Geometry: final body of the model. Coordinates: model frame, mm. Face numbers are marked on the shaded views. A direction names the side the tool comes from. Coordinates: 2 decimals unless noted, no trailing zeros. Loops run counter-clockwise (first coordinate to the right, second up) from the corner with the lowest first, then second, coordinate; pieces in that order, holes last. Notation, with made-up numbers: (-39.75, 38.25) - (-33.75, 38.25) arc R18 ccw to (-33.75, 73.25) - close; hole circle Ø6 at (80.5, -7.5). An arc over 180 degrees is marked (long way). Answer in a Markdown table with one row per item.
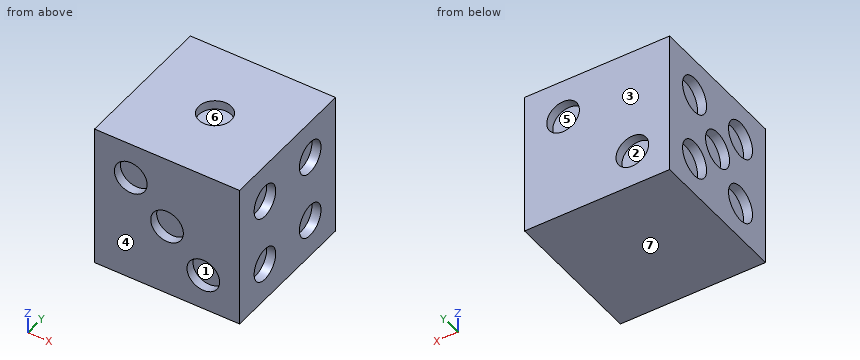
Autodesk Fusion 360 part; units mm, degrees
sketch "Sketch1" plane through (0, 0, 0) normal (0, 0, 1) x (1, 0, 0) in component "Component"
  line L0 (50.8, -50.8) -> (-50.8, -50.8)
  line L1 (-50.8, -50.8) -> (-50.8, 50.8)
  line L2 (-50.8, 50.8) -> (50.8, 50.8)
  line L3 (50.8, 50.8) -> (50.8, -50.8)
  line L4 (50.8, -50.8) -> (-50.8, 50.8) construction
  line L5 (-50.8, -50.8) -> (50.8, 50.8) construction
  dimension "d1" = 101.6
  dimension "d2" = 101.6
extrude "Extrude1" add sketch "Sketch1" along normal mid plane 101.6 in component "Component"
sketch "Sketch2" plane through (0, 0, 50.8) normal (0, 0, 1) x (-1, 0, 0) in component "Component"
  line L0 (-50.8, -50.8) -> (50.8, -50.8)
  line L1 (50.8, -50.8) -> (50.8, 50.8)
  line L2 (50.8, 50.8) -> (-50.8, 50.8)
  line L3 (-50.8, 50.8) -> (-50.8, -50.8)
  circle A0 centre (0, 0) radius 11.43
  dimension "d5" = 22.86
extrude "Extrude2" cut sketch "Sketch2" against normal blind 6.35 contours A0 in component "Component"
sketch "Sketch3" plane through (0, -50.8, 0) normal (0, -1, 0) x (1, 0, 0) in component "Component"
  line L0 (50.8, -50.8) -> (50.8, 50.8)
  line L1 (50.8, 50.8) -> (-50.8, 50.8)
  line L2 (-50.8, 50.8) -> (-50.8, -50.8)
  line L3 (-50.8, -50.8) -> (50.8, -50.8)
  circle A0 centre (0, 0) radius 11.43
  line L4 (-50.8, 50.8) -> (0, 0)
  line L5 (0, 0) -> (50.8, -50.8)
  circle A1 centre (-25.4, 25.4) radius 11.43
  circle A2 centre (25.4, -25.4) radius 11.43
  dimension "d8" = 22.86
  dimension "d9" = 22.86
  dimension "d10" = 22.86
extrude "Extrude3" cut sketch "Sketch3" against normal blind 6.35 contours L5 A2 | L5 A2 | L4 A1 | L4 A1 | A0 L4 L5 | A0 L4 L5 in component "Component"
sketch "Sketch4" plane through (50.8, 0, 0) normal (1, 0, 0) x (0, 1, 0) in component "Component"
  line L0 (50.8, -50.8) -> (50.8, 50.8)
  line L1 (50.8, 50.8) -> (-50.8, 50.8)
  line L2 (-50.8, 50.8) -> (-50.8, -50.8)
  line L3 (-50.8, -50.8) -> (50.8, -50.8)
  line L4 (-50.8, 50.8) -> (50.8, -50.8)
  line L5 (-50.8, -50.8) -> (50.8, 50.8) construction
  circle A0 centre (-23.9624, 23.9624) radius 11.43
  circle A1 centre (23.9624, 23.9624) radius 11.43
  circle A2 centre (-23.9624, -23.9624) radius 11.43
  circle A3 centre (23.9624, -23.9624) radius 11.43
  dimension "d13" = 22.86
extrude "Extrude4" cut sketch "Sketch4" against normal blind 6.35 contours L4 A3 | L4 A3 | L4 A0 | L4 A0 | A1 | A2 in component "Component"
sketch "Sketch5" plane through (0, 50.8, 0) normal (0, 1, 0) x (-1, 0, 0) in component "Component"
  line L0 (50.8, -50.8) -> (50.8, 50.8)
  line L1 (50.8, 50.8) -> (-50.8, 50.8)
  line L2 (-50.8, 50.8) -> (-50.8, -50.8)
  line L3 (-50.8, -50.8) -> (50.8, -50.8)
  line L4 (-50.8, 50.8) -> (50.8, -50.8)
  circle A0 centre (24.6983, -24.6983) radius 11.43
  circle A1 centre (-23.7784, 23.7784) radius 11.43
  dimension "d16" = 22.86
extrude "Extrude5" cut sketch "Sketch5" against normal blind 6.35 contours L4 A0 | L4 A0 | L4 A1 | L4 A1 in component "Component"
sketch "Sketch6" plane through (-50.8, 0, 0) normal (-1, 0, 0) x (0, -1, 0) in component "Component"
  line L0 (50.8, -50.8) -> (50.8, 50.8)
  line L1 (50.8, 50.8) -> (-50.8, 50.8)
  line L2 (-50.8, 50.8) -> (-50.8, -50.8)
  line L3 (-50.8, -50.8) -> (50.8, -50.8)
  line L4 (-50.8, 50.8) -> (50.8, -50.8)
  line L5 (-50.8, -50.8) -> (50.8, 50.8)
  circle A0 centre (0, 0) radius 12.7
  circle A1 centre (-24.3304, 24.3304) radius 12.7
  circle A2 centre (24.3304, 24.3304) radius 12.7
  circle A3 centre (-24.3304, -24.3304) radius 12.7
  circle A4 centre (24.3304, -24.3304) radius 12.7
  dimension "d19" = 25.4
extrude "Extrude6" cut sketch "Sketch6" against normal blind 6.35 contours L4 A4 | L4 A4 | L5 A2 | L5 A2 | L5 A3 | L5 A3 | L4 A1 | L4 A1 | L4 L5 A0 | L4 L5 A0 | L4 L5 A0 | L4 L5 A0 in component "Component"
sketch "Sketch7" plane through (0, 0, -50.8) normal (0, 0, -1) x (1, 0, 0) in component "Component"
  line L0 (-50.8, -50.8) -> (50.8, -50.8)
  line L1 (50.8, -50.8) -> (50.8, 50.8)
  line L2 (50.8, 50.8) -> (-50.8, 50.8)
  line L3 (-50.8, 50.8) -> (-50.8, -50.8)
sketch "Sketch8" plane through (0, 50.8, 0) normal (0, 1, 0) x (-1, 0, 0) in component "Component"
  circle A0 centre (24.6983, -24.6983) radius 11.43
  circle A1 centre (-23.7784, 23.7784) radius 11.43
  line L0 (50.8, -50.8) -> (50.8, 50.8)
  line L1 (50.8, 50.8) -> (-50.8, 50.8)
  line L2 (-50.8, 50.8) -> (-50.8, -50.8)
  line L3 (-50.8, -50.8) -> (50.8, -50.8)
sketch "Sketch10" plane through (0, 0, -50.8) normal (0, 0, -1) x (1, 0, 0) in component "Component"
component "Component" placed x (1, 0, 0) y (0, 1, 0) z (0, 0, 1) at (0, 0, 0)
equation "d1 = dicesize"
equation "d2 = dicesize"
equation "d5 = Divotsize"
equation "d8 = Divotsize"
equation "d9 = Divotsize"
equation "d10 = Divotsize"
equation "d13 = Divotsize"
equation "d16 = Divotsize"
equation "dicesize = 4 in"
equation "Divotsize = 0.9 in"
equation "diceDepth = 0.25 in"
(1) Pull-direction query (Z, two-part tool) for the marked faces 4, 5, 6 and 7; classes: pulls with the +Z half, pulls with the -Z half, needs draft (parallel to the pull), parting line crosses it, or undercut.
Verdict:
| item | result |
|---|---|
| face 4 | needs draft |
| face 5 | undercut |
| face 6 | pulls with the +Z half |
| face 7 | pulls with the -Z half |
(2) Cut plane A-A on y = 0. Output: boundary loops of the cut face in (x, z), then the cut area to 3 significant figures.
Verdict:
| item | result |
|---|---|
| outline | (-50.8, -50.8) - (50.8, -50.8) - (50.8, 50.8) - (11.43, 50.8) - (11.43, 44.45) - (-11.43, 44.45) - (-11.43, 50.8) - (-50.8, 50.8) - (-50.8, 12.7) - (-44.45, 12.7) - (-44.45, -12.7) - (-50.8, -12.7) - close |
| area | 10,000 mm² |
(3) Cut plane D-D on z = 20.5. Output: boundary loops of the cut face in (x, y), then the cut area to 3 significant figures.
Verdict:
| item | result |
|---|---|
| outline | (-50.8, -50.8) - (-35.73, -50.8) - (-35.73, -44.45) - (-15.07, -44.45) - (-15.07, -50.8) - (50.8, -50.8) - (50.8, -34.86) - (44.45, -34.86) - (44.45, -13.07) - (50.8, -13.07) - (50.8, 13.07) - (44.45, 13.07) - (44.45, 34.86) - (50.8, 34.86) - (50.8, 50.8) - (34.73, 50.8) - (34.73, 44.45) - (12.83, 44.45) - (12.83, 50.8) - (-50.8, 50.8) - (-50.8, 36.44) - (-44.45, 36.44) - (-44.45, 12.22) - (-50.8, 12.22) - (-50.8, -12.22) - (-44.45, -12.22) - (-44.45, -36.44) - (-50.8, -36.44) - close |
| area | 9,470 mm² |
(4) First-contact query: pin 1 Ø13.5 at (y, z) = (-23.96, 23.96) entering from +X; pin 2 Ø1.5 at (y, z) = (-3.5, -1) entering from -X; pin 3 Ø20.5 at (x, y) = (0, 0) entering from +Z. Flat tips, straight axial feed; report the tip coordinate or a pass-through.
Verdict:
| item | result |
|---|---|
| pin 1 | stops at x = 44.45 |
| pin 2 | stops at x = -44.45 |
| pin 3 | stops at z = 44.45 |
(5) Access query for the marked faces 1, 2 and 3. Directions: +Z, -Z, +X, -X, +Y, -Y. A direction counts if a zero-diameter tool reaches every point of the face in a straight line with its end or side. Return the directions, or none.
Verdict:
| item | result |
|---|---|
| face 1 | -Y |
| face 2 | +Y |
| face 3 | +Z, -Z, +X, -X, +Y |
(6) Ray query, probe 1 along Y at (x, z) = (-47, 0); probe 2 along X at (y, z) = (-47.75, 0); probe 3 along X at (y, z) = (-29, 21.5). Return the intervals inside material, ascending.
Verdict:
| item | result |
|---|---|
| probe 1 | y = -50.8 to -12.7, 12.7 to 50.8 |
| probe 2 | x = -50.8 to -11.43, 11.43 to 50.8 |
| probe 3 | x = -44.45 to 44.45 |
(7) Cut plane C-C on z = -32.5. Output: boundary loops of the cut face in (x, y).
Verdict:
| item | result |
|---|---|
| outline | (-50.8, -50.8) - (16.44, -50.8) - (16.44, -44.45) - (34.36, -44.45) - (34.36, -50.8) - (50.8, -50.8) - (50.8, -31.56) - (44.45, -31.56) - (44.45, -16.36) - (50.8, -16.36) - (50.8, 16.36) - (44.45, 16.36) - (44.45, 31.56) - (50.8, 31.56) - (50.8, 50.8) - (-16.34, 50.8) - (-16.34, 44.45) - (-33.05, 44.45) - (-33.05, 50.8) - (-50.8, 50.8) - (-50.8, 34.05) - (-44.45, 34.05) - (-44.45, 14.61) - (-50.8, 14.61) - (-50.8, -14.61) - (-44.45, -14.61) - (-44.45, -34.05) - (-50.8, -34.05) - close |
(8) Cut plane B-B on x = 0. Output: boundary loops of the cut face in (y, z), then the cut area to 3 significant figures.
Verdict:
| item | result |
|---|---|
| outline | (-50.8, -50.8) - (50.8, -50.8) - (50.8, 50.8) - (11.43, 50.8) - (11.43, 44.45) - (-11.43, 44.45) - (-11.43, 50.8) - (-50.8, 50.8) - (-50.8, 11.43) - (-44.45, 11.43) - (-44.45, -11.43) - (-50.8, -11.43) - close |
| area | 10,000 mm² |
